Here's how the part is built. I have some questions about the finished solid (model axes, mm). A direction names the side the tool comes from. Give positions to 0.01 mm unless a question says otherwise; leave off trailing zeros. Order: outer loops, then holes, each group sorted by start corner. A loop starts at its lowest first (then second) coordinate and runs counter-clockwise, first axis right, second up. Notation, with made-up numbers: (-37.75, -3.75) -> (-6.75, -3.75) arc R10 ccw to (-6.75, 5.25) -> close; hole circle Ø9 at (77.25, 29). An arc over 180 degrees is marked (long way). Write each question's results on one line, items separated by ' | '. Start each with the question number.
Q1. For faces 4 (the face through (2, 0, -26)), 5 (the face through (0, 15, -80)), which set-ups out of +Z, -Z, +X, -X, +Y, -Y let a thin tool reach every point of the face, with its end or its side?
Q2. I need wall thicknesses on line 1 along Z through (x, y) = (0, 17.75); line 2 along Z through (x, y) = (0, 11.75); line 3 along Y through (x, z) = (102.5, -8). Which ranges of each line are inside material? Lowest first, please. Write a range as [from, to].
Q3. Imagine slicing it at A-A, the plane z = 0. Please give me the cut outline in (x, y), then the cut area to 3 significant figures.
Q4. Imagine slicing it at D-D, the plane x = -80. Please give me the cut outline in (y, z), then the cut area to 3 significant figures.
Q5. I'm going to push flat-ended pins straight in: pin 1 (25 mm diameter, centred on x = -3, z = 73, fed in from +Y); pin 2 (8 mm diameter, centred on y = 8.5, z = -81, fed in from -X); pin 3 (1 mm diameter, centred on x = 33.5, y = 16, fed in from +Z). Where does each tip first touch, or does it pass through?
Q6. Imagine slicing it at B-B, the plane x = 0. Please give me the cut outline in (y, z), then the cut area to 3 significant figures.
Q7. Thinking about a two-plate mould opening in X: for faces 1 (the face through (124.88, 9.86, -5.5)), 2 (the face through (2, 20, -26)), 3 (the face through (23.846, 10.14, -7.509)), which applies, pulls with the +X half, pulls with the -X half, needs draft (parallel to the pull), parting line crosses it, or undercut?
Q8. Imagine slicing it at C-C, the plane y = 9.5. Please give me the cut outline in (x, z), then the cut area to 3 significant figures.
Autodesk Inventor part; units mm, degrees
ref_plane "YZ Plane" through (0, 0, 0) normal (1, 0, 0) x (0, 1, 0)
ref_plane "XZ Plane" through (0, 0, 0) normal (0, 1, 0) x (-1, 0, 0)
ref_plane "XY Plane" through (0, 0, 0) normal (0, 0, 1) x (1, 0, 0)
sketch "Sketch1" plane through (0, 0, 0) normal (0, 1, 0) x (-1, 0, 0)
  point P0 (0, 0)
extrude "Extrusion1" [suppressed]
sketch "Sketch2" plane through (0, 0, 0) normal (0, 1, 0) x (-1, 0, 0)
  circle A0 centre (0, 0) radius 125
  dimension "d3" = 250
extrude "Extrusion2" add sketch "Sketch2" along normal blind 20
sketch "Sketch3" plane through (0, 20, 0) normal (0, 1, 0) x (1, 0, 0)
  circle A0 centre (0, 0) radius 25
  dimension "d6" = 50
extrude "Extrusion3" cut sketch "Sketch3" against normal blind 20
sketch "Sketch4" plane through (0, 20, 0) normal (0, 1, 0) x (1, 0, 0)
  line L0 (0, 0) -> (0, 80)
  circle A0 centre (0, 80) radius 25
  dimension "d9" = 80
  dimension "d10" = 50
extrude "Extrusion4" cut sketch "Sketch4" against normal blind 5
sketch "Sketch5" plane through (0, 20, 0) normal (0, 1, 0) x (1, 0, 0)
  line L0 (0, 0) -> (80, 0)
  circle A0 centre (80, 0) radius 25
  dimension "d13" = 80
  dimension "d14" = 50
extrude "Extrusion5" cut sketch "Sketch5" against normal blind 5
sketch "Sketch6" plane through (0, 20, 0) normal (0, 1, 0) x (1, 0, 0)
  line L0 (0, 0) -> (-80, 0)
  circle A0 centre (-80, 0) radius 25
  dimension "d17" = 80
  dimension "d18" = 50
extrude "Extrusion6" cut sketch "Sketch6" against normal blind 5
sketch "Sketch7" plane through (0, 20, 0) normal (0, 1, 0) x (1, 0, 0)
  line L0 (0, 0) -> (0, -80)
  circle A0 centre (0, -80) radius 25
  dimension "d21" = 80
  dimension "d22" = 50
extrude "Extrusion7" cut sketch "Sketch7" against normal blind 5
properties part number "expo12"
Geometry check:
1) face 4: +Z, -Z, +X, -X, -Y | face 5: +Y
2) line 1: [-125, -105], [-55, -25], [25, 55], [105, 125] | line 2: [-125, -25], [25, 125] | line 3: [0, 15]
3) outline: (-125, 0) -> (-25, 0) -> (-25, 20) -> (-55, 20) -> (-55, 15) -> (-105, 15) -> (-105, 20) -> (-125, 20) -> close; (25, 0) -> (125, 0) -> (125, 20) -> (105, 20) -> (105, 15) -> (55, 15) -> (55, 20) -> (25, 20) -> close | area: 3,500 mm²
4) outline: (0, -96.05) -> (20, -96.05) -> (20, -25) -> (15, -25) -> (15, 25) -> (20, 25) -> (20, 96.05) -> (0, 96.05) -> close | area: 3,590 mm²
5) pin 1: y = 15 | pin 2: x = -98.47 | pin 3: z = 120.57
6) outline: (0, -125) -> (20, -125) -> (20, -105) -> (15, -105) -> (15, -55) -> (20, -55) -> (20, -25) -> (0, -25) -> close; (0, 25) -> (20, 25) -> (20, 55) -> (15, 55) -> (15, 105) -> (20, 105) -> (20, 125) -> (0, 125) -> close | area: 3,500 mm²
7) face 1: parting line crosses it | face 2: needs draft | face 3: undercut
8) outline: circle Ø250 at (0, 0); hole circle Ø50 at (0, 0) | area: 47,100 mm²
